Build history of the part. All positions in model axes, mm. Face numbers are marked on the shaded views. A direction names the side the tool comes from. Round coordinates to 2 decimals unless told otherwise and drop trailing zeros. Write each loop counter-clockwise with the first axis right and the second up, starting at its lowest first coordinate (ties: lowest second). Pieces come first, ordered by that corner, then holes. Notation, with made-up numbers: M 66,40 L 103,40 A20 ccw 103,51 Z; hole C 57.25,-21.5 d2. An arc over 180 degrees is marked long. Write item = value, one per line.
from build123d import *

# Parameters (mm, degrees)
SKETCH1_W           = 127
SKETCH1_H           = 63.5
BOSS_EXTRUDE1_DEPTH = 25.4
SKETCH2_R           = 6.858
CUT_EXTRUDE1_DEPTH  = 19.05
SKETCH3_R           = 6.858
CUT_EXTRUDE2_DEPTH  = 19.05


with BuildPart() as part:
    # Sketch1 → Boss-Extrude1 (new body)
    with BuildSketch(Plane(origin=(0, 0, 0), x_dir=(1, 0, 0), z_dir=(0, 1, 0))):
        Rectangle(SKETCH1_W, SKETCH1_H)
    extrude(amount=BOSS_EXTRUDE1_DEPTH)

    # Sketch2 → Cut-Extrude1 (cut)
    with BuildSketch(Plane.XY.offset(31.75)):
        with Locations((0, 12.7)):
            Circle(SKETCH2_R)
    extrude(amount=-CUT_EXTRUDE1_DEPTH, mode=Mode.SUBTRACT)

    # Sketch3 → Cut-Extrude2 (cut)
    with BuildSketch(Plane(origin=(0, 0, -31.75), x_dir=(-1, 0, 0), z_dir=(0, 0, -1))):
        with Locations((25.4, 12.7)):
            Circle(SKETCH3_R)
        with Locations((-25.4, 12.7)):
            Circle(SKETCH3_R)
    extrude(amount=-CUT_EXTRUDE2_DEPTH, mode=Mode.SUBTRACT)


solid = part.part
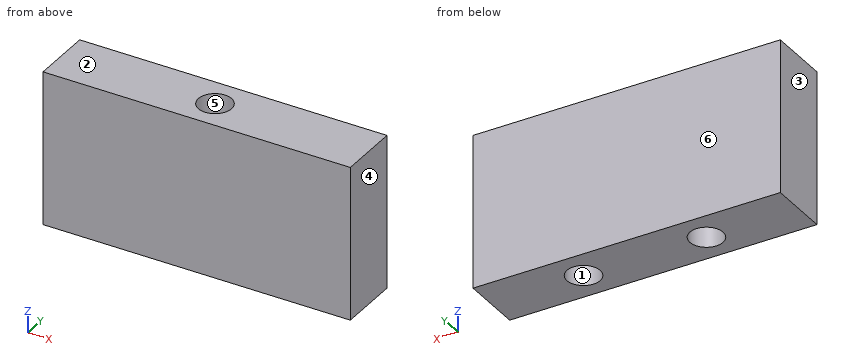
1. Mould opens along X. For the marked faces 3, 4, 5 and 6 say: pulls with the +X half, pulls with the -X half, needs draft (parallel to the pull), parting line crosses it, or undercut.
Responses:
face_3 = pulls with the -X half
face_4 = pulls with the +X half
face_5 = undercut
face_6 = needs draft
2. Band-saw the part on C-C (x = 21). List the corners of the cut face in (y, z), plus the area to 3 significant figures.
Responses:
outline = M 0,-31.75 L 7.44,-31.75 L 7.44,-12.7 L 17.96,-12.7 L 17.96,-31.75 L 25.4,-31.75 L 25.4,31.75 L 0,31.75 Z
area = 1,410 mm²
3. Tool access for the marked faces 1 and 2: list every direction of +Z, -Z, +X, -X, +Y, -Y with a clear straight run to the whole face (end or side of a thin tool).
Responses:
face_1 = -Z
face_2 = +Z, +X, -X, +Y, -Y
4. Probe probe 1 along X at (y, z) = (10, -26); probe 2 along Y at (x, z) = (0, 24); probe 3 along X at (y, z) = (17, -21.5). List the from-to ranges inside material, lowest first.
Responses:
probe_1 = -63.5 to -31.7, -19.1 to 19.1, 31.7 to 63.5
probe_2 = 0 to 5.84, 19.56 to 25.4
probe_3 = -63.5 to -30.74, -20.06 to 20.06, 30.74 to 63.5
5. Flat gauge pins, fed straight in: pin 1 (7 mm diameter, centred on x = 1.5, y = 12.5, fed in from +Z); pin 2 (7 mm diameter, centred on x = -26, y = 10.5, fed in from -Z). Where does each tip first touch, or does it go through?
Responses:
pin_1 = 12.7
pin_2 = -12.7
6. Band-saw the part on A-A (x = -25.4). List the corners of the cut face in (y, z), plus the area to 3 significant figures.
Responses:
outline = M 0,-31.75 L 5.84,-31.75 L 5.84,-12.7 L 19.56,-12.7 L 19.56,-31.75 L 25.4,-31.75 L 25.4,31.75 L 0,31.75 Z
area = 1,350 mm²
7. Band-saw the part on B-B (y = 12.7). List the corners of the cut face in (x, z).
Responses:
outline = M -63.5,-31.75 L -32.26,-31.75 L -32.26,-12.7 L -18.54,-12.7 L -18.54,-31.75 L 18.54,-31.75 L 18.54,-12.7 L 32.26,-12.7 L 32.26,-31.75 L 63.5,-31.75 L 63.5,31.75 L 6.86,31.75 L 6.86,12.7 L -6.86,12.7 L -6.86,31.75 L -63.5,31.75 Z
